The figure shows three views and two pictorial views of one solid part (mm, origin at its lowest corner). Answer the questions. Round coordinates to 2 decimals unless told otherwise and drop trailing zeros. Order: outer loops, then holes, each group sorted by start corner. A loop starts at its lowest first (then second) coordinate and runs counter-clockwise, first axis right, second up. Notation, with made-up numbers: M 74.5,66 L 132.5,66 A28 cw 132.5,90 Z; hole C -35.5,43 d8. An arc over 180 degrees is marked long. Return JSON: item names as keys, results as strings.
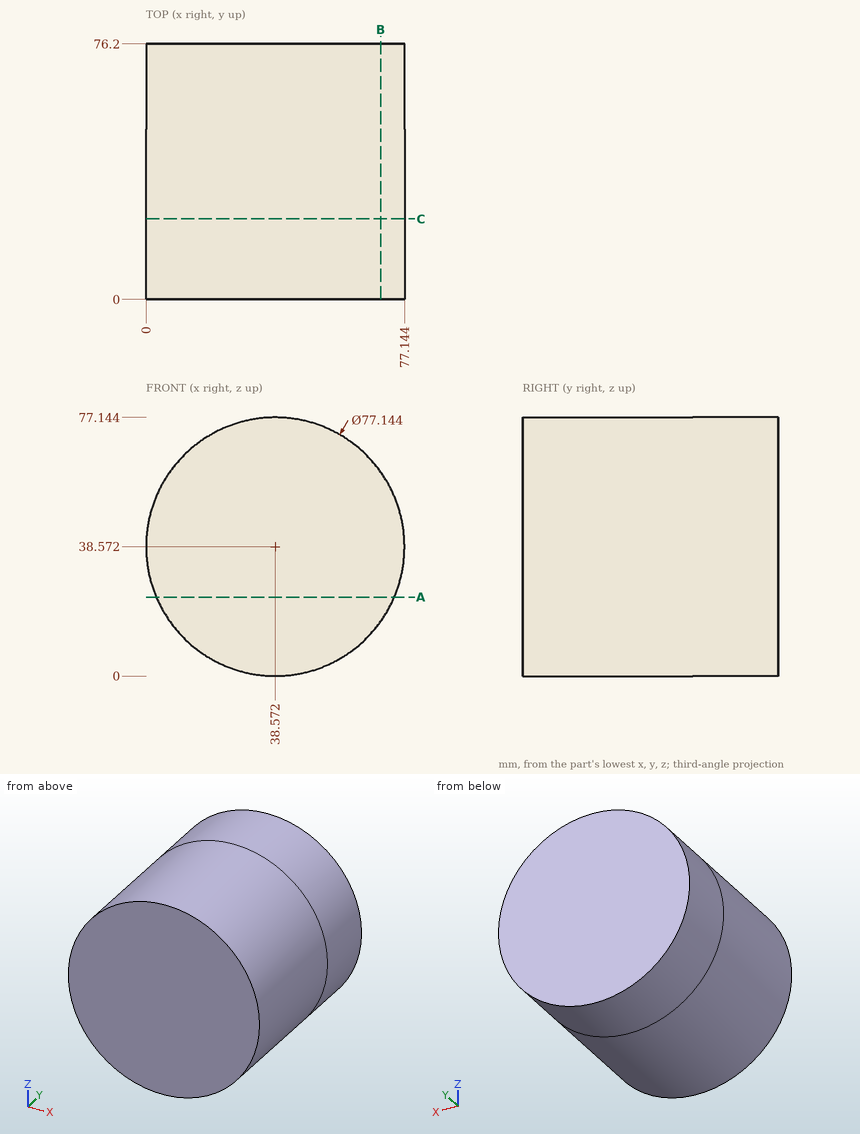
Item 1: Consider line 1 along Z through (x, y) = (44, 55) (1 decimal); line 2 along X through (y, z) = (34.5, 24) (1 decimal). Determine where each line is inside the solid, lowest interval first. Write a range as [from, to].
Output:
{"line 1": "z = [0.4, 76.8]", "line 2": "x = [2.9, 74.3]"}
Item 2: Find section B-B (x = 70). Determine the outline of the cut face in (y, z) (1 decimal), plus the area to 3 significant figures.
Output:
{"outline": "M 0,16.2 L 76.2,16.2 L 76.2,60.9 L 0,60.9 Z", "area": "3,410 mm^2"}
Item 3: Find section C-C (y = 24). Determine the outline of the cut face in (x, z) (1 decimal), plus the area to 3 significant figures.
Output:
{"outline": "C 38.6,38.6 d77.1", "area": "4,670 mm^2"}
Item 4: Each of these flat-tipped pins is pushed along its axis until it touches: pin 1 (12 mm diameter, centred on y = 39.5, z = 50.5, fed in from +X); pin 2 (10 mm diameter, centred on x = 13.5, z = 38.5, fed in from -Y); pin 3 (12 mm diameter, centred on y = 11, z = 66, fed in from +X) (1 decimal); pin 4 (6 mm diameter, centred on y = 55, z = 27.5, fed in from +X). Where does it stop, or does it pass through?
Output:
{"pin 1": "stops at x = 76.69", "pin 2": "stops at y = 0", "pin 3": "stops at x = 70.6", "pin 4": "stops at x = 76.29"}
Item 5: Find section A-A (z = 23.5). Determine the outline of the cut face in (x, y).
Output:
{"outline": "M 3.07,0 L 74.08,0 L 74.08,76.2 L 3.07,76.2 Z"}
